```python
from build123d import *

# Parameters (mm, degrees)
SKETCH_1_W          = 160
SKETCH_1_H          = 80
EXTRUDE_1_DEPTH     = 14.5
SKETCH_3_R          = 2
CUT_EXTRUDE_1_DEPTH = 10


with BuildPart() as part:
    # 草图1 → 凸台-拉伸1 (new body)
    with BuildSketch(Plane(origin=(0, 0, 0), x_dir=(1, 0, 0), z_dir=(0, 1, 0))):
        with Locations((0, 40)):
            Rectangle(SKETCH_1_W, SKETCH_1_H)
    extrude(amount=EXTRUDE_1_DEPTH)

    # 草图3 → 切除-拉伸1 (cut)
    with BuildSketch(Plane.XZ):
        with Locations(Location((-30, -15, 0), (0, 0, 270))):
            Circle(SKETCH_3_R)
        with Locations(Location((30, -15, 0), (0, 0, 270))):
            Circle(SKETCH_3_R)
    extrude(amount=-CUT_EXTRUDE_1_DEPTH, mode=Mode.SUBTRACT)


solid = part.part
```
Geometry check sheet. Reference: the model listing, model coordinates, mm. A direction names the side the tool comes from. Give positions to 0.01 mm unless a question says otherwise; leave off trailing zeros. Write each loop counter-clockwise with the first axis right and the second up, starting at its lowest first coordinate (ties: lowest second). Pieces come first, ordered by that corner, then holes. Notation, with made-up numbers: (36, 5) - (94, 5) arc R14 ccw to (94, 20) - close; hole circle Ø6 at (-23.5, -24.5). An arc over 180 degrees is marked (long way). Use a Markdown table: item, result.
Q1. Section check B-B, the plane x = -30. Enter the section's corners in (y, z), then the cut area to 3 significant figures.
Computed:
| item | result |
|---|---|
| outline | (0, -80) - (14.5, -80) - (14.5, 0) - (0, 0) - (0, -13) - (10, -13) - (10, -17) - (0, -17) - close |
| area | 1,120 mm² |
Q2. Section check A-A, the plane z = -15. Enter the section's corners in (x, y), then the cut area to 3 significant figures.
Computed:
| item | result |
|---|---|
| outline | (-80, 0) - (-32, 0) - (-32, 10) - (-28, 10) - (-28, 0) - (28, 0) - (28, 10) - (32, 10) - (32, 0) - (80, 0) - (80, 14.5) - (-80, 14.5) - close |
| area | 2,240 mm² |
Q3. Go/stop test with a flat-tipped pin: P1, Ø3.5, axis at x = -30, z = -15, coming from the -Y side. Record where the tip stops, or that it passes through.
Computed:
| item | result |
|---|---|
| P1 | stops at y = 10 |
Q4. Set-up check for faces 5 (the face through (28, 5, -15)), 6 (the face through (-1, 7, 0)): record each of +Z, -Z, +X, -X, +Y, -Y from which the full face is reachable in a straight line by a thin tool's end or side.
Computed:
| item | result |
|---|---|
| face 5 | -Y |
| face 6 | +Z, +X, -X, +Y, -Y |
Q5. Draft check along X on faces 1 (the face through (-1, 14.5, -41)), 2 (the face through (-80, 7, -39)), 3 (the face through (80, 7, -39)), 4 (the face through (-32, 5, -15)). Enter one of: pulls with the +X half, pulls with the -X half, needs draft (parallel to the pull), parting line crosses it, or undercut.
Computed:
| item | result |
|---|---|
| face 1 | needs draft |
| face 2 | pulls with the -X half |
| face 3 | pulls with the +X half |
| face 4 | undercut |
Q6. Thickness scan on L1, parallel to X at y = 4, z = -15; L2, parallel to X at y = 1, z = -13.5; L3, parallel to Z at x = 30.5, y = 9. Record the ranges inside material, lowest first. Write a range as [from, to].
Computed:
| item | result |
|---|---|
| L1 | x = [-80, -32], [-28, 28], [32, 80] |
| L2 | x = [-80, -31.32], [-28.68, 28.68], [31.32, 80] |
| L3 | z = [-80, -16.94], [-13.06, 0] |
